For this review, use the dimensioned drawing (mm, ordinates from the lowest corner) and the shaded views. Round coordinates to 2 decimals unless told otherwise and drop trailing zeros. Loops run counter-clockwise (first coordinate to the right, second up) from the corner with the lowest first, then second, coordinate; pieces in that order, holes last. Notation, with made-up numbers: M -22.75,13.5 L 1.25,13.5 A24 ccw 1.25,23.5 Z; hole C 86.25,82 d5. An arc over 180 degrees is marked long. Write item = value, one per line. Start each with the question number.
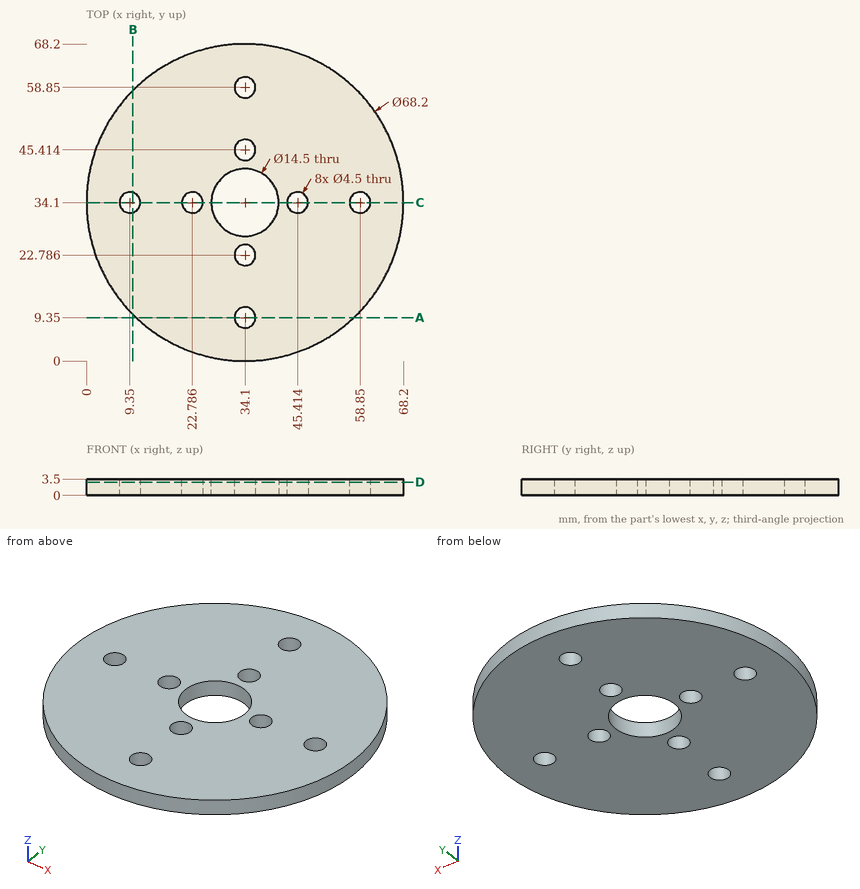
(1) For pin 1 Ø1.5 at (y, z) = (12.5, 2) entering from +X, flat-tipped, find the tip position at first contact; note if it passes through.
(2) Add section C-C on y = 34.1. Write out the cut boundary in (x, z), and give its area (3 significant figures).
(3) Add section B-B on x = 10. Write out the cut boundary in (y, z) (1 decimal), and give its area (3 significant figures).
(4) Add section D-D on z = 2.8. Count the separate pieces of the cut face and the enclosed holes in it, and give its area (3 significant figures).
(5) Wall thickness on L1, parallel to Y at x = 34.1, z = 1.5; L2, parallel to X at y = 47, z = 1.3 (1 decimal); L3, parallel to X at y = 10.5, z = 3 (1 decimal): over which ranges is each line inside the solid? List them lowest first.
(6) Add section A-A on y = 9.35. Write out the cut boundary in (x, z).
Answer sheet:
q1.pin_1 = 61.08
q2.outline = M 0,0 L 7.1,0 L 7.1,3.5 L 0,3.5 Z; M 11.6,0 L 20.54,0 L 20.54,3.5 L 11.6,3.5 Z; M 25.04,0 L 26.85,0 L 26.85,3.5 L 25.04,3.5 Z; M 41.35,0 L 43.16,0 L 43.16,3.5 L 41.35,3.5 Z; M 47.66,0 L 56.6,0 L 56.6,3.5 L 47.66,3.5 Z; M 61.1,0 L 68.2,0 L 68.2,3.5 L 61.1,3.5 Z
q2.area = 125 mm²
q3.outline = M 10,0 L 31.9,0 L 31.9,3.5 L 10,3.5 Z; M 36.3,0 L 58.2,0 L 58.2,3.5 L 36.3,3.5 Z
q3.area = 154 mm²
q4.separate_pieces = 1
q4.enclosed_holes = 9
q4.area = 3,360 mm²
q5.L1 = 0 to 7.1, 11.6 to 20.54, 25.04 to 26.85, 41.35 to 43.16, 47.66 to 56.6, 61.1 to 68.2
q5.L2 = 2.5 to 32.5, 35.7 to 65.7
q5.L3 = 9.5 to 32.2, 36 to 58.7
q6.outline = M 10.64,0 L 31.85,0 L 31.85,3.5 L 10.64,3.5 Z; M 36.35,0 L 57.56,0 L 57.56,3.5 L 36.35,3.5 Z
